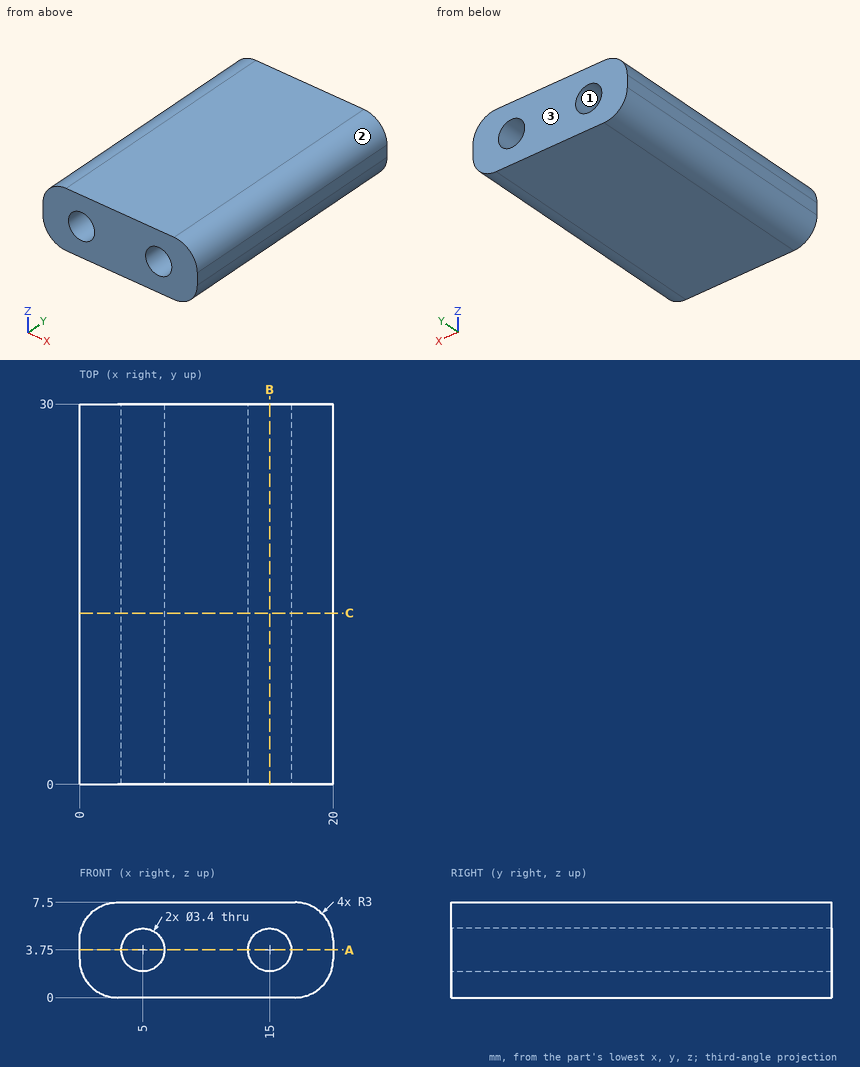
Geometry: see drawing. Coordinates: mm, zero at the bounding-box minimum. Give positions to 0.01 mm unless a question says otherwise; leave off trailing zeros. Loops run counter-clockwise (first coordinate to the right, second up) from the corner with the lowest first, then second, coordinate; pieces in that order, holes last. Notation, with made-up numbers: (52.5, 70) - (79.5, 70) arc R32 ccw to (79.5, 104) - close; hole circle Ø2 at (73, 9). An arc over 180 degrees is marked (long way). Use CSV: the item, a comma, the result in double quotes.
1) Cut plane C-C (y = 13.5). Output: boundary loops of the cut face in (x, z).
Worked out:
outline,"(0, 3) arc R3 ccw to (3, 0) - (17, 0) arc R3 ccw to (20, 3) - (20, 4.5) arc R3 ccw to (17, 7.5) - (3, 7.5) arc R3 ccw to (0, 4.5) - close; hole circle Ø3.4 at (5, 3.75); hole circle Ø3.4 at (15, 3.75)"
2) Mould query, pull axis X, two halves, no side actions, for the marked faces 1, 2 and 3. Classes: +X half, -X half, draft (parallel to the pull), parting line (faces both ways), or undercut.
Worked out:
face 1,"undercut"
face 2,"+X half"
face 3,"draft"
3) Cut plane B-B (x = 15). Output: boundary loops of the cut face in (y, z).
Worked out:
outline,"(0, 0) - (30, 0) - (30, 2.05) - (0, 2.05) - close; (0, 5.45) - (30, 5.45) - (30, 7.5) - (0, 7.5) - close"
4) Cut plane A-A (z = 3.75). Output: boundary loops of the cut face in (x, y), and give its area (3 significant figures).
Worked out:
outline,"(0, 0) - (3.3, 0) - (3.3, 30) - (0, 30) - close; (6.7, 0) - (13.3, 0) - (13.3, 30) - (6.7, 30) - close; (16.7, 0) - (20, 0) - (20, 30) - (16.7, 30) - close"
area,"396 mm^2"
5) Pin query (flat end, axial travel): P1, Ø1.5, axis at x = 5.5, z = 5, coming from the -Y side; P2, Ø1, axis at y = 23, z = 6, coming from the -X side. Return the tip coordinate at first contact, or that it passes through.
Worked out:
P1,"stops at y = 0"
P2,"stops at x = 0.17"
6) Line query: line 1 (Z direction, x = 5, y = 11.5); line 2 (X direction, y = 15.5, z = 2.5); line 3 (Z direction, x = 4, y = 3.5). Output: solid intervals per line, ascending.
Worked out:
line 1,"z = 0 to 2.05, 5.45 to 7.5"
line 2,"x = 0.04 to 3.85, 6.15 to 13.85, 16.15 to 19.96"
line 3,"z = 0 to 2.38, 5.12 to 7.5"
